Read the model definition and answer for the solid it produces. Units are mm, in the model's axes. Coordinates: 2 decimals unless noted, no trailing zeros. Loops run counter-clockwise (first coordinate to the right, second up) from the corner with the lowest first, then second, coordinate; pieces in that order, holes last.
Autodesk Inventor part; units mm, degrees
ref_plane "YZ Plane" through (0, 0, 0) normal (1, 0, 0) x (0, 1, 0)
ref_plane "XZ Plane" through (0, 0, 0) normal (0, 1, 0) x (-1, 0, 0)
ref_plane "XY Plane" through (0, 0, 0) normal (0, 0, 1) x (1, 0, 0)
sketch "Sketch1" plane through (0, 0, 0) normal (0, 0, 1) x (1, 0, 0)
  line L0 (-2.7678, 3.3517) -> (22.6322, 3.3517)
  line L1 (22.6322, 3.3517) -> (22.6322, -47.4483)
  line L2 (22.6322, -47.4483) -> (-2.7678, -47.4483)
  line L3 (-2.7678, -47.4483) -> (-2.7678, 3.3517)
  line L4 (19.5061, 0.2256) -> (0.3583, 0.2256)
  line L5 (0.3583, 0.2256) -> (0.3583, -44.3222)
  line L6 (0.3583, -44.3222) -> (19.5061, -44.3222)
  line L7 (19.5061, -44.3222) -> (19.5061, 0.2256)
  point P0 (0, 0)
  dimension "d0" = 25.4
  dimension "d1" = 50.8
extrude "Extrusion1" add sketch "Sketch1" along normal blind 1016
sketch "Sketch2" plane through (-2.7678, 3.3517, 0) normal (0, 1, 0) x (1, 0, 0)
  point P0 (2.7678, 0)
properties part number "40in 2x1 boxbeam"
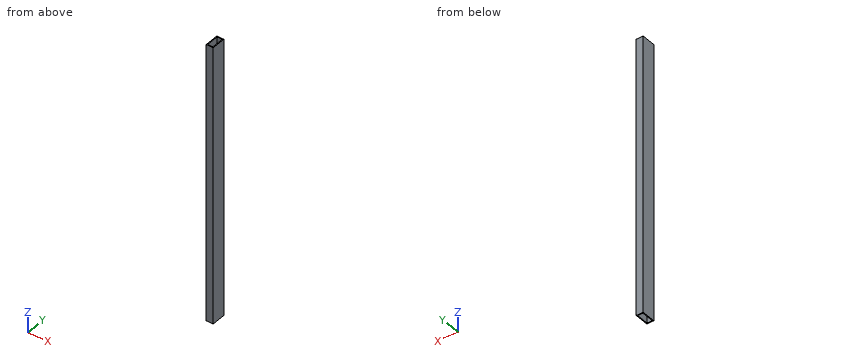
Q1. Straight lines are drawn through the part: probe 1 along X at (y, z) = (-18, 326.5); probe 2 along Y at (x, z) = (11.25, 300.5). For each, find the intervals that lie inside material, in ascending order.
Findings below:
probe 1: x = -2.77 to 0.36, 19.51 to 22.63
probe 2: y = -47.45 to -44.32, 0.23 to 3.35
Q2. A cutting plane is placed at C-C (x = 4.75). Give the vertices of the cut face in (y, z), then the cut area to 3 significant figures.
Findings below:
outline: (-47.45, 0) - (-44.32, 0) - (-44.32, 1016) - (-47.45, 1016) - close; (0.23, 0) - (3.35, 0) - (3.35, 1016) - (0.23, 1016) - close
area: 6,350 mm2
Q3. A cutting plane is placed at B-B (z = 349). Give the vertices of the cut face in (x, y), then the cut area to 3 significant figures.
Findings below:
outline: (-2.77, -47.45) - (22.63, -47.45) - (22.63, 3.35) - (-2.77, 3.35) - close; hole (0.36, -44.32) - (19.51, -44.32) - (19.51, 0.23) - (0.36, 0.23) - close
area: 437 mm2
Q4. A flat-ended cylindrical pin translates along its axis: pin 1 Ø12 at (x, y) = (1.5, -17.5) entering from -Z. Find the tip coordinate at first contact, or state that the pin passes through.
Findings below:
pin 1: stops at z = 0
Q5. A cutting plane is placed at A-A (y = -8.5). Give the vertices of the cut face in (x, z).
Findings below:
outline: (-2.77, 0) - (0.36, 0) - (0.36, 1016) - (-2.77, 1016) - close; (19.51, 0) - (22.63, 0) - (22.63, 1016) - (19.51, 1016) - close
